Read the model definition and answer for the solid it produces. Units are mm, in the model's axes. A direction names the side the tool comes from. Round coordinates to 2 decimals unless told otherwise and drop trailing zeros. Order: outer loops, then holes, each group sorted by start corner. A loop starts at its lowest first (then second) coordinate and runs counter-clockwise, first axis right, second up.
from build123d import *

# Parameters (mm, degrees)
SKETCH1_W                                        = 40.64
SKETCH1_H                                        = 40.64
BOSS_EXTRUDE1_DEPTH                              = 7.62
SKETCH2_W                                        = 4.318
SKETCH2_H                                        = 40.64
BOSS_EXTRUDE2_DEPTH                              = 10.16
F_10_CLEARANCE_HOLE1_D                           = 5.1054
CBORE_FOR_1_4_BUTTON_HEAD_CAP_SCREW1_D           = 6.7564
CBORE_FOR_1_4_BUTTON_HEAD_CAP_SCREW1_CBORE_D     = 11.90752
CBORE_FOR_1_4_BUTTON_HEAD_CAP_SCREW1_CBORE_DEPTH = 3.3528
CUT_EXTRUDE1_REACH                               = 62.161
SKETCH8_R                                        = 7.965368028
FILLET1_R                                        = 4.572


with BuildPart() as part:
    # Sketch1 → Boss-Extrude1 (new body)
    with BuildSketch(Plane(origin=(0, 0, 0), x_dir=(1, 0, 0), z_dir=(0, 1, 0))):
        with Locations((20.32, -20.32)):
            Rectangle(SKETCH1_W, SKETCH1_H)
    extrude(amount=BOSS_EXTRUDE1_DEPTH)

    # Sketch2 → Boss-Extrude2 (add)
    with BuildSketch(Plane(origin=(0, 7.62, 0), x_dir=(1, 0, 0), z_dir=(0, 1, 0))):
        with Locations((2.159, -20.32)):
            Rectangle(SKETCH2_W, SKETCH2_H)
        with Locations((38.481, -20.32)):
            Rectangle(SKETCH2_W, SKETCH2_H)
    extrude(amount=BOSS_EXTRUDE2_DEPTH)

    # #10 Clearance Hole1 (through all)
    with Locations(Plane.ZY):
        with Locations((9.144, 12.319), (31.496, 12.319)):
            Hole(F_10_CLEARANCE_HOLE1_D / 2)

    # CBORE for 1/4 Button Head Cap Screw1 (through all)
    with Locations(Plane(origin=(0, 7.62, 0), x_dir=(1, 0, 0), z_dir=(0, 1, 0))):
        with Locations((12.7, -6.985), (12.7, -33.655)):
            CounterBoreHole(CBORE_FOR_1_4_BUTTON_HEAD_CAP_SCREW1_D / 2, CBORE_FOR_1_4_BUTTON_HEAD_CAP_SCREW1_CBORE_D / 2, CBORE_FOR_1_4_BUTTON_HEAD_CAP_SCREW1_CBORE_DEPTH)

    # Sketch8 → Cut-Extrude1 (cut, up to next)
    with BuildSketch(Plane(origin=(40.64, 0, 0), x_dir=(0, 0, -1), z_dir=(1, 0, 0)), mode=Mode.PRIVATE) as cut_extrude1_sk1:
        with Locations((-20.32, 19.504553012)):
            Circle(SKETCH8_R)
    cut_extrude1_tool1 = extrude(cut_extrude1_sk1.sketch, amount=-CUT_EXTRUDE1_REACH, mode=Mode.PRIVATE) & part.part
    add(cut_extrude1_tool1.solids().sort_by_distance((40.64, 19.504553, 20.32))[0], mode=Mode.SUBTRACT)

    # Fillet1
    fillet1_edges = [part.edges().sort_by_distance(p)[0] for p in [
        (2.159, 17.78, 40.64),
        (2.159, 17.78, 0),
        (38.481, 17.78, 40.64),
        (38.481, 17.78, 0),
        (38.481, 17.78, 28.096439078),
        (38.481, 17.78, 12.543560922),
    ]]
    fillet(fillet1_edges, radius=FILLET1_R)


solid = part.part
Q1. A cutting plane is placed at D-D, the plane y = 3.75. Give the vertices of the cut face in (x, z) (3 decimals), plus the area to 3 significant figures.
Outcome:
outline: (0, 0) - (40.64, 0) - (40.64, 40.64) - (0, 40.64) - close; hole circle Ø6.756 at (12.7, 6.985); hole circle Ø6.756 at (12.7, 33.655)
area: 1,580 mm2
Q2. Straight lines are drawn through the part: probe 1 along Z at (x, y) = (12.7, 2.4); probe 2 along X at (y, z) = (9.25, 18); probe 3 along Y at (x, z) = (35.5, 11). For each, find the intervals that lie inside material, in ascending order.
Outcome:
probe 1: z = 0 to 3.61, 10.36 to 30.28, 37.03 to 40.64
probe 2: x = 0 to 4.32, 36.32 to 40.64
probe 3: y = 0 to 7.62
Q3. A cutting plane is placed at B-B, the plane x = 12.7. Give the vertices of the cut face in (y, z), plus the area to 3 significant figures.
Outcome:
outline: (0, 0) - (7.62, 0) - (7.62, 1.03) - (4.27, 1.03) - (4.27, 3.61) - (0, 3.61) - close; (0, 10.36) - (4.27, 10.36) - (4.27, 12.94) - (7.62, 12.94) - (7.62, 27.7) - (4.27, 27.7) - (4.27, 30.28) - (0, 30.28) - close; (0, 37.03) - (4.27, 37.03) - (4.27, 39.61) - (7.62, 39.61) - (7.62, 40.64) - (0, 40.64) - close
area: 172 mm2
Q4. For a pull along X with two mould halves and no side action, classify faces 6 (the face through (15.3, 4.267, 36.2)), 7 (the face through (2.2, 16.5, 1.4)), 8 (the face through (0, 9, 21)), 9 (the face through (18.38, 5.97, 5.2)) as released by +X, released by -X, zero draft, split by the parting line, or undercut.
Outcome:
face 6: undercut
face 7: zero draft
face 8: released by -X
face 9: undercut
Q5. A cutting plane is placed at A-A, the plane y = 8.5. Give the vertices of the cut face in (x, z).
Outcome:
outline: (0, 0) - (4.32, 0) - (4.32, 40.64) - (0, 40.64) - close; (36.32, 0) - (40.64, 0) - (40.64, 40.64) - (36.32, 40.64) - close
Q6. For faces 1 (the face through (4.318, 13, 21)), 2 (the face through (15, 4.267, 10)), 3 (the face through (38.511, 17.187, 28.91)), 4 (the face through (38, 17.78, 34)), 5 (the face through (38.511, 12.431, 34.046)), determine the directions among +Z, -Z, +X, -X, +Y, -Y from which every point of the face is accessible in a straight line to the end or side of a thin tool.
Outcome:
face 1: +Z, -Z, +Y
face 2: +Y
face 3: +X, +Y
face 4: +Z, -Z, +X, -X, +Y
face 5: +X, -X
Q7. Flat-ended cylindrical pins translate along their axes: pin 1 (8 mm diameter, centred on y = 12.319, z = 31.496, fed in from +X); pin 2 (9.5 mm diameter, centred on x = 22.5, z = 19.5, fed in from +Y). Find the tip coordinate at first contact, or state that the pin passes through.
Outcome:
pin 1: stops at x = 40.64
pin 2: stops at y = 7.62
Q8. A cutting plane is placed at C-C, the plane z = 8. Give the vertices of the cut face in (x, y).
Outcome:
outline: (0, 0) - (9.48, 0) - (9.48, 4.27) - (6.83, 4.27) - (6.83, 7.62) - (4.32, 7.62) - (4.32, 10.04) - (0, 10.04) - close; (0, 14.6) - (4.32, 14.6) - (4.32, 17.78) - (0, 17.78) - close; (15.92, 0) - (40.64, 0) - (40.64, 10.04) - (36.32, 10.04) - (36.32, 7.62) - (18.57, 7.62) - (18.57, 4.27) - (15.92, 4.27) - close; (36.32, 14.6) - (40.64, 14.6) - (40.64, 17.78) - (36.32, 17.78) - close
